Part model, mm, in its own coordinate system. Face numbers are marked on the shaded views. A direction names the side the tool comes from. Give positions to 0.01 mm unless a question says otherwise; leave off trailing zeros. Write each loop counter-clockwise with the first axis right and the second up, starting at its lowest first coordinate (ties: lowest second). Pieces come first, ordered by that corner, then holes. Notation, with made-up numbers: (58.25, 32) - (117.25, 32) arc R20 cw to (117.25, 57) - close; hole circle Ø3 at (49.25, -10). An arc over 180 degrees is marked (long way). Answer as a JSON object with one key per item and string values. Group by question number.
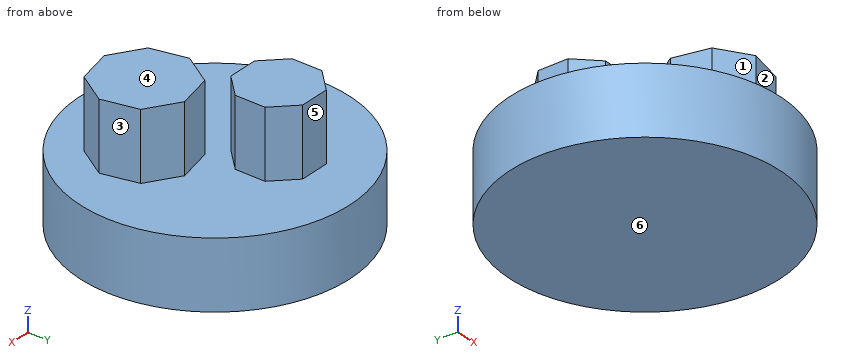
```python
from build123d import *

# Parameters (mm, degrees)
F0_R     = 50
F1_DEPTH = 25
F3_DEPTH = 25


with BuildPart() as f1:
    # F0 (on Top) → F1 (new body)
    with BuildSketch(Plane.XY):
        Circle(F0_R)
    extrude(amount=F1_DEPTH)

    # F2 (on face) → F3 (join)
    with BuildSketch(Plane.XY.offset(25)):
        Polygon((3.619255, -0.923771), (-3.619255, -12.274176), (-0.711706, -25.418523), (10.638699, -32.657032), (23.783046, -29.749483), (31.021555, -18.399078), (28.114006, -5.254732), (16.763601, 1.983778), align=None)
        Polygon((-3.070575, 30.081054), (-14.102733, 30.081054), (-21.903647, 22.28014), (-21.903647, 11.247983), (-14.102733, 3.447069), (-3.070575, 3.447069), (4.730338, 11.247983), (4.730338, 22.28014), align=None)
    extrude(amount=F3_DEPTH)


solid = f1.part
```
1) Saw through at B-B (y = 13.5). List the corners of the cut face in (x, z).
2) Saw through at C-C (x = 6). List the corners of the cut face in (y, z), and give its area (3 significant figures).
3) Drill centre lines: line 1 along Z through (x, y) = (39, -14); line 2 along X through (y, z) = (18, 38); line 3 along Y through (x, z) = (0, 3). Where is each one in solid material? Low to high. Write a range as from..to.
4) Saw through at D-D (z = 16.5). List the corners of the cut face in (x, y), and give its area (3 significant figures).
5) Two-plate mould, pull along Z, no slides. Class the marked faces 4, 5 and 6: +Z half, -Z half, draft (parallel to the pull), parting line (faces both ways), or undercut.
6) Drop flat-ended pins along their axis: P1, Ø10, axis at y = -20, z = 12.5, coming from the -X side; P2, Ø1, axis at x = 36.5, z = 23.5, coming from the +Y side; P3, Ø3.5, axis at y = 16, z = 35, coming from the +X side. Give the stop position or say it passes through.
7) Which spindle directions (+Z, -Z, +X, -X, +Y, -Y) get a long thin tool onto all of the face, cutting with end or side? Do the marked faces 1, 2 and 3. Say none if no direction does.
8) Saw through at A-A (z = 35.5). List the corners of the cut face in (x, y), and give its area (3 significant figures).
Checks:
{
 "1": {"outline": "(-48.14, 0) - (48.14, 0) - (48.14, 25) - (4.73, 25) - (4.73, 50) - (-21.9, 50) - (-21.9, 25) - (-48.14, 25) - close"},
 "2": {"outline": "(-49.64, 0) - (49.64, 0) - (49.64, 25) - (-0.4, 25) - (-0.4, 50) - (-29.7, 50) - (-29.7, 25) - (-49.64, 25) - close", "area": "3,210 mm2"},
 "3": {"line 1": "0..25", "line 2": "-21.9..4.73", "line 3": "-50..50"},
 "4": {"outline": "circle Ø100 at (0, 0)", "area": "7,850 mm2"},
 "5": {"face 4": "+Z half", "face 5": "draft", "face 6": "-Z half"},
 "6": {"P1": "x = -47.7", "P2": "y = 34.7", "P3": "x = 4.73"},
 "7": {"face 1": "+Z, -X, -Y", "face 2": "+Z, +X, -Y", "face 3": "+Z, +X, +Y"},
 "8": {"outline": "(-21.9, 11.25) - (-14.1, 3.45) - (-3.07, 3.45) - (4.73, 11.25) - (4.73, 22.28) - (-3.07, 30.08) - (-14.1, 30.08) - (-21.9, 22.28) - close; (-3.62, -12.27) - (-0.71, -25.42) - (10.64, -32.66) - (23.78, -29.75) - (31.02, -18.4) - (28.11, -5.25) - (16.76, 1.98) - (3.62, -0.92) - close", "area": "1,460 mm2"}
}
